Part model, mm, in its own coordinate system. A direction names the side the tool comes from. Coordinates: 2 decimals unless noted, no trailing zeros. Loops run counter-clockwise (first coordinate to the right, second up) from the corner with the lowest first, then second, coordinate; pieces in that order, holes last. Notation, with made-up numbers: (-27.75, 33.25) - (19.25, 33.25) arc R21 cw to (19.25, 59.25) - close; hole circle Ø1 at (-11.75, 86.5). An arc over 180 degrees is marked (long way). Answer as CSV lines item,"result".
from build123d import *

# Parameters (mm, degrees)
ESQUISSE1_R        = 12.5
ESQUISSE1_R_2      = 5
ESQUISSE1_R_3      = 0.75
BOSS_EXTRU_1_DEPTH = 2
ESQUISSE2_R        = 12.5
ESQUISSE2_R_2      = 10.5
BOSS_EXTRU_2_DEPTH = 3


with BuildPart() as part:
    # Esquisse1 → Boss.-Extru.1 (new body)
    with BuildSketch(Plane.XY):
        Circle(ESQUISSE1_R)
        Circle(ESQUISSE1_R_2, mode=Mode.SUBTRACT)
        with Locations((-5.25, 5.25)):
            Circle(ESQUISSE1_R_3, mode=Mode.SUBTRACT)
        with Locations((5.25, 5.25)):
            Circle(ESQUISSE1_R_3, mode=Mode.SUBTRACT)
        with Locations((5.25, -5.25)):
            Circle(ESQUISSE1_R_3, mode=Mode.SUBTRACT)
        with Locations((-5.25, -5.25)):
            Circle(ESQUISSE1_R_3, mode=Mode.SUBTRACT)
    extrude(amount=BOSS_EXTRU_1_DEPTH)

    # Esquisse2 → Boss.-Extru.2 (add)
    with BuildSketch(Plane.XY.offset(2)):
        Circle(ESQUISSE2_R)
        Circle(ESQUISSE2_R_2, mode=Mode.SUBTRACT)
    extrude(amount=BOSS_EXTRU_2_DEPTH)


solid = part.part
Q1. Saw through at A-A (x = 0). Give the cut face in (y, z).
Results:
outline,"(-12.5, 0) - (-5, 0) - (-5, 2) - (-10.5, 2) - (-10.5, 5) - (-12.5, 5) - close; (5, 0) - (12.5, 0) - (12.5, 5) - (10.5, 5) - (10.5, 2) - (5, 2) - close"
Q2. Which spindle directions (+Z, -Z, +X, -X, +Y, -Y) get a long thin tool onto all of the face, cutting with end or side? Do faces 4 (the face through (10, 3.2, 3.5)), 5 (the face through (4.5, 5.3, 1)). Say none if no direction does.
Results:
face 4,"+Z"
face 5,"+Z, -Z"
Q3. Saw through at C-C (z = 1.25). Give the cut face in (x, y).
Results:
outline,"circle Ø25 at (0, 0); hole circle Ø1.5 at (-5.25, -5.25); hole circle Ø1.5 at (-5.25, 5.25); hole circle Ø10 at (0, 0); hole circle Ø1.5 at (5.25, -5.25); hole circle Ø1.5 at (5.25, 5.25)"
Q4. Wall check: L1, parallel to Z at x = -8, y = 6.25; L2, parallel to Y at x = 0, z = 0.95; L3, parallel to X at y = 7.5, z = 2.55. Give the ranges that are in metal, low to high.
Results:
L1,"z = 0 to 2"
L2,"y = -12.5 to -5, 5 to 12.5"
L3,"x = -10 to -7.35, 7.35 to 10"
Q5. Saw through at D-D (x = 8.75). Give the cut face in (y, z).
Results:
outline,"(-8.93, 0) - (8.93, 0) - (8.93, 5) - (5.8, 5) - (5.8, 2) - (-5.8, 2) - (-5.8, 5) - (-8.93, 5) - close"
Q6. Flat gauge pins, fed straight in: pin 1 (2 mm diameter, centred on x = -5.25, y = 5.25, fed in from +Z); pin 2 (3 mm diameter, centred on x = 3.5, z = 3, fed in from +Y); pin 3 (1 mm diameter, centred on y = -1, z = 3, fed in from -X). Where does each tip first touch, or does it go through?
Results:
pin 1,"stops at z = 2"
pin 2,"stops at y = 12.34"
pin 3,"stops at x = -12.49"
Q7. Two-plate mould, pull along X, no slides. Class faces 1 (the face through (11.923, 3.755, 2.465)), 2 (the face through (-5.845, -5.706, 0.986)), 3 (the face through (-0.2, -5.4, 0)): released by +X, released by -X, zero draft, split by the parting line, or undercut.
Results:
face 1,"split by the parting line"
face 2,"undercut"
face 3,"zero draft"
